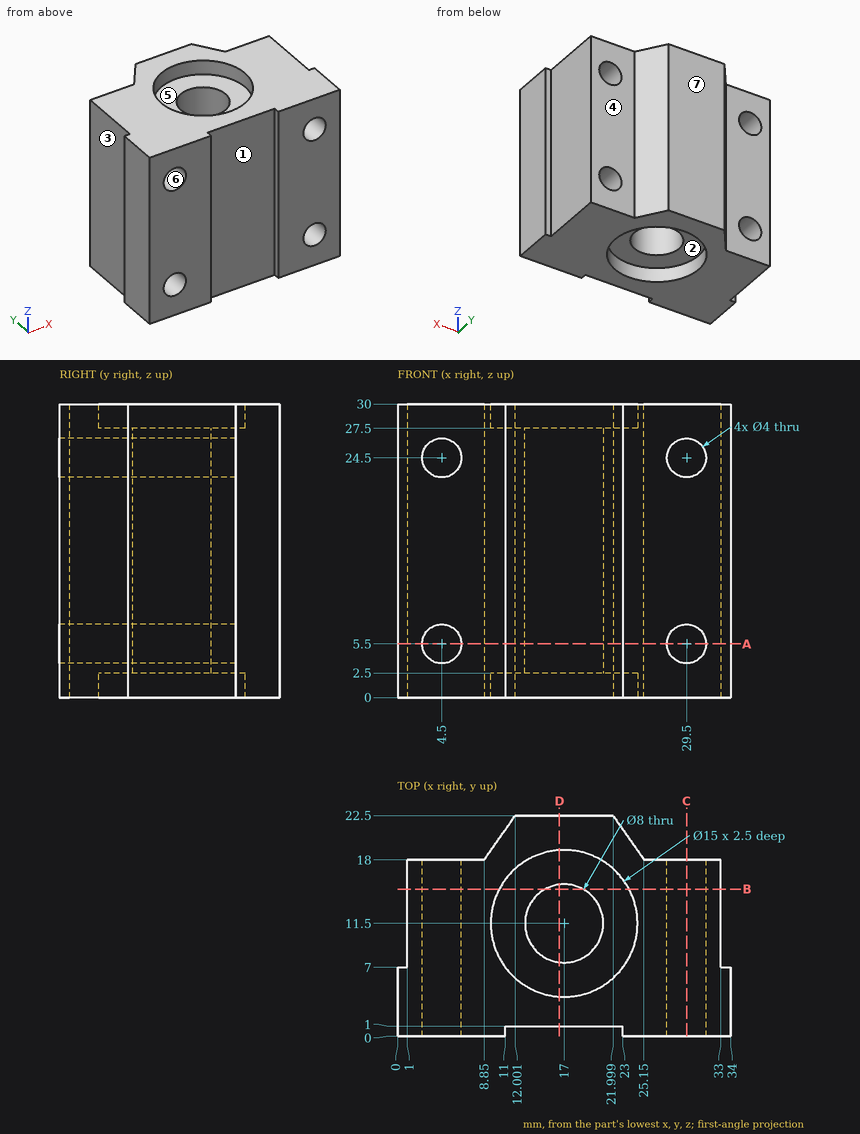
Geometry check sheet. Reference: drawing and pictorial views, mm from the part's lowest x, y, z. A direction names the side the tool comes from. Round coordinates to 2 decimals unless told otherwise and drop trailing zeros. Loops run counter-clockwise (first coordinate to the right, second up) from the corner with the lowest first, then second, coordinate; pieces in that order, holes last. Notation, with made-up numbers: M 58.5,23.25 L 109.5,23.25 A21 ccw 109.5,33.25 Z; hole C 72,-16.75 d1. An arc over 180 degrees is marked long. Return JSON: item names as keys, results as strings. Group by question number.
(1) Set-up check for the marked faces 1, 2, 3 and 4: record each of +Z, -Z, +X, -X, +Y, -Y from which the full face is reachable in a straight line by a thin tool's end or side.
(2) Mould release check, pull along Y, two halves, no side actions. Record for the marked faces 5, 6 and 7: pulls with the +Y half, pulls with the -Y half, needs draft (parallel to the pull), parting line crosses it, or undercut.
(3) Section check D-D, the plane x = 16.5. Enter the section's corners in (y, z).
(4) Section check A-A, the plane z = 5.5. Enter the section's corners in (x, y).
(5) Go/stop test with flat-tipped pins: pin 1 (6.5 mm diameter, centred on x = 5, z = 20, fed in from +Y); pin 2 (13.5 mm diameter, centred on x = 17, y = 11.5, fed in from +Z); pin 3 (9 mm diameter, centred on y = 14.5, z = 15.5, fed in from +X). Record where each tip stops, or that it passes through.
(6) Scan lines: line 1 along Z through (x, y) = (4.5, 5.5); line 2 along X through (y, z) = (5.75, 24.5); line 3 along Z through (x, y) = (3.5, 10). Record each from-to range of solid material in increasing order. Write a range as [from, to].
(7) Section check C-C, the plane x = 29.5. Enter the section's corners in (y, z), and give its area (3 significant figures).
(8) Section check B-B, the plane y = 15. Enter the section's corners in (x, z), and give its area (3 significant figures).
Data:
{
 "1": {"face 1": "+Z, -Z, -Y", "face 2": "-Z", "face 3": "+Z, -Z, -X, +Y", "face 4": "+Z, -Z, +X, +Y"},
 "2": {"face 5": "undercut", "face 6": "needs draft", "face 7": "pulls with the +Y half"},
 "3": {"outline": "M 1,0 L 4.02,0 L 4.02,2.5 L 7.53,2.5 L 7.53,27.5 L 4.02,27.5 L 4.02,30 L 1,30 Z; M 15.47,2.5 L 18.98,2.5 L 18.98,0 L 22.5,0 L 22.5,30 L 18.98,30 L 18.98,27.5 L 15.47,27.5 Z"},
 "4": {"outline": "M 0,0 L 2.5,0 L 2.5,18 L 1,18 L 1,7 L 0,7 Z; M 6.5,0 L 11,0 L 11,1 L 23,1 L 23,0 L 27.5,0 L 27.5,18 L 25.15,18 L 22,22.5 L 12,22.5 L 8.85,18 L 6.5,18 Z; M 31.5,0 L 34,0 L 34,7 L 33,7 L 33,18 L 31.5,18 Z; hole C 17,11.5 d8"},
 "5": {"pin 1": "y = 18", "pin 2": "z = 27.5", "pin 3": "x = 33"},
 "6": {"line 1": "[0, 3.5], [7.5, 22.5], [26.5, 30]", "line 2": "[0, 2.5], [6.5, 27.5], [31.5, 34]", "line 3": "[0, 3.77], [7.23, 22.77], [26.23, 30]"},
 "7": {"outline": "M 0,0 L 18,0 L 18,3.5 L 0,3.5 Z; M 0,7.5 L 18,7.5 L 18,22.5 L 0,22.5 Z; M 0,26.5 L 18,26.5 L 18,30 L 0,30 Z", "area": "396 mm²"},
 "8": {"outline": "M 1,0 L 10.37,0 L 10.37,2.5 L 15.06,2.5 L 15.06,27.5 L 10.37,27.5 L 10.37,30 L 1,30 Z; M 18.94,2.5 L 23.63,2.5 L 23.63,0 L 33,0 L 33,30 L 23.63,30 L 23.63,27.5 L 18.94,27.5 Z; hole C 4.5,5.5 d4; hole C 4.5,24.5 d4; hole C 29.5,5.5 d4; hole C 29.5,24.5 d4", "area": "747 mm²"}
}
